```python
from build123d import *

# Parameters (mm, degrees)
CYLINDER001_R           = 7.5
CYLINDER001_DEPTH       = 50
CYLINDER003_R           = 11
CYLINDER003_DEPTH       = 7.1
CYLINDER002_R           = 11
CYLINDER002_DEPTH       = 7.1
CYLINDER004_R           = 3.95
CYLINDER004_DEPTH       = 48
CYLINDER004_PITCH_ANGLE = 90
CYLINDER_R              = 12.5
CYLINDER_DEPTH          = 21


with BuildPart() as cylindre001:
    # Cylinder001 → Cylinder001 (new body)
    with BuildSketch(Plane.XY.offset(-11)):
        Circle(CYLINDER001_R)
    extrude(amount=CYLINDER001_DEPTH)


with BuildPart() as cylindre003:
    # Cylinder003 → Cylinder003 (new body)
    with BuildSketch(Plane.XY.offset(13.91)):
        Circle(CYLINDER003_R)
    extrude(amount=CYLINDER003_DEPTH)


with BuildPart() as cylindre002:
    # Cylinder002 → Cylinder002 (new body)
    with BuildSketch(Plane.XY.offset(-0.0001)):
        Circle(CYLINDER002_R)
    extrude(amount=CYLINDER002_DEPTH)


with BuildPart() as axe_rotation:
    # Cylinder004 → Cylinder004 (new body)
    with BuildSketch(Plane.XY):
        Circle(CYLINDER004_R)
    extrude(amount=CYLINDER004_DEPTH)


with BuildPart() as axe_rotation_1:
    # Cylinder004 pitch: moved
    add(axe_rotation.part.rotate(Axis((0, 0, 0), (0, 1, 0)), CYLINDER004_PITCH_ANGLE))


with BuildPart() as axe_rotation_2:
    # Cylinder004 placement: moved
    add(axe_rotation_1.part.moved(Location((-23, 0, 10.5))))


with BuildPart() as obj1:
    # Cylinder → Cylinder (new body)
    with BuildSketch(Plane.XY):
        Circle(CYLINDER_R)
    extrude(amount=CYLINDER_DEPTH)

    # Fusion: union Axe rotation
    add(axe_rotation_2.part)

    # Cut003: cut Cylindre002
    add(cylindre002.part, mode=Mode.SUBTRACT)

    # Cut004: cut Cylindre003
    add(cylindre003.part, mode=Mode.SUBTRACT)

    # Cut005: cut Cylindre001
    add(cylindre001.part, mode=Mode.SUBTRACT)


solid = obj1.part
```
For this review, take the finished solid that the model builds, in its own axes (mm). A direction names the side the tool comes from. Coordinates: 2 decimals unless noted, no trailing zeros. Write each loop counter-clockwise with the first axis right and the second up, starting at its lowest first coordinate (ties: lowest second). Pieces come first, ordered by that corner, then holes. Notation, with made-up numbers: (53, -27) - (71, -27) arc R37 ccw to (71, 11) - close; hole circle Ø3 at (60, 50). An arc over 180 degrees is marked (long way). Put each result on its own line as item: value.
1. Machinability: for faces 4 (the cylindrical face through (-17.508, 0.174, 14.446)), 5 (the cylindrical face through (18.338, 1.186, 6.732)), 6 (the flat face through (7.2, 2.6, 13.91)), which of the approach directions +Z, -Z, +X, -X, +Y, -Y give a long, thin tool a straight path to every point of the face, cutting with its end or side? Answer none if there is none.
Values found:
face 4: -X
face 5: +X
face 6: +Z
2. Wall thickness on probe 1 along Y at (x, z) = (0, 15.5); probe 2 along Y at (x, z) = (0, 9.75): over which ranges is each line inside the solid? List them lowest first.
Values found:
probe 1: -12.5 to -11, 11 to 12.5
probe 2: -12.5 to -7.5, 7.5 to 12.5
3. Add section B-B, the plane x = 0. Give the boundary of the cut face in (y, z).
Values found:
outline: (-12.5, 0) - (-11, 0) - (-11, 7.1) - (-7.5, 7.1) - (-7.5, 13.91) - (-11, 13.91) - (-11, 21) - (-12.5, 21) - close; (7.5, 7.1) - (11, 7.1) - (11, 0) - (12.5, 0) - (12.5, 21) - (11, 21) - (11, 13.91) - (7.5, 13.91) - close
4. Add section C-C, the plane z = 10.5. Give the boundary of the cut face in (x, y), then the cut area to 3 significant figures.
Values found:
outline: (-23, -3.95) - (-11.86, -3.95) arc R12.5 ccw to (11.86, -3.95) - (25, -3.95) - (25, 3.95) - (11.86, 3.95) arc R12.5 ccw to (-11.86, 3.95) - (-23, 3.95) - close; hole circle Ø15 at (0, 0)
area: 499 mm²
5. Mouldability with a two-part tool opening along X and no side actions: class faces 1 (the cylindrical face through (11.547, -4.788, 10.353)), 2 (the flat face through (5, -10, 0)), 3 (the flat face through (7.2, 2.6, 7.1)) as released by +X, released by -X, zero draft, split by the parting line, or undercut.
Values found:
face 1: split by the parting line
face 2: zero draft
face 3: undercut
6. Add section D-D, the plane y = 3.25. Give the boundary of the cut face in (x, z) (3 decimals), then the cut area to 3 significant figures.
Values found:
outline: (-23, 8.255) - (-12.07, 8.255) - (-12.07, 0) - (-10.509, 0) - (-10.509, 7.1) - (-6.759, 7.1) - (-6.759, 13.91) - (-10.509, 13.91) - (-10.509, 21) - (-12.07, 21) - (-12.07, 12.745) - (-23, 12.745) - close; (6.759, 7.1) - (10.509, 7.1) - (10.509, 0) - (12.07, 0) - (12.07, 8.255) - (25, 8.255) - (25, 12.745) - (12.07, 12.745) - (12.07, 21) - (10.509, 21) - (10.509, 13.91) - (6.759, 13.91) - close
area: 224 mm²
7. For pin 1 (8 mm diameter, centred on x = 17, z = 10.5, fed in from +Y); pin 2 (9 mm diameter, centred on x = 0, y = 0, fed in from -Z); pin 3 (5 mm diameter, centred on x = -15.5, y = -5.5, fed in from -Z); pin 4 (4 mm diameter, centred on y = 9, z = 14.5, fed in from +X), all flat-tipped, find the tip position at first contact; note any pin that passes through.
Values found:
pin 1: y = 3.95
pin 2: through
pin 3: z = 7.93
pin 4: x = 10.36
8. Add section A-A, the plane y = 0. Give the boundary of the cut face in (x, z), then the cut area to 3 significant figures.
Values found:
outline: (-23, 6.55) - (-12.5, 6.55) - (-12.5, 0) - (-11, 0) - (-11, 7.1) - (-7.5, 7.1) - (-7.5, 13.91) - (-11, 13.91) - (-11, 21) - (-12.5, 21) - (-12.5, 14.45) - (-23, 14.45) - close; (7.5, 7.1) - (11, 7.1) - (11, 0) - (12.5, 0) - (12.5, 6.55) - (25, 6.55) - (25, 14.45) - (12.5, 14.45) - (12.5, 21) - (11, 21) - (11, 13.91) - (7.5, 13.91) - close
area: 292 mm²
